Verification items for the finished model (mm, model axes). Face numbers are marked on the shaded views. Coordinates: 2 decimals unless noted, no trailing zeros. Order: outer loops, then holes, each group sorted by start corner. A loop starts at its lowest first (then second) coordinate and runs counter-clockwise, first axis right, second up. Notation, with made-up numbers: M 32.5,-1.75 L 83.5,-1.75 A21 ccw 83.5,15.25 Z; hole C 34,-37 d3. An arc over 180 degrees is marked long. Write item = value, one per line.
```python
from build123d import *

# Parameters (mm, degrees)
EXTRUDE_1_DEPTH     = 8
SKETCH_2_R          = 7.5
CUT_EXTRUDE_1_DEPTH = 10


with BuildPart() as part:
    # 草图1 → 凸台-拉伸1 (new body)
    with BuildSketch(Plane(origin=(0, 0, 0), x_dir=(0, 0, -1), z_dir=(1, 0, 0))):
        with BuildLine():
            ThreePointArc((15, 0), (0, 15), (-15, 0))
            Line((-15, 0), (-12.5, -200))
            ThreePointArc((-12.5, -200), (0, -212.5), (12.5, -200))
            Line((12.5, -200), (15, 0))
        make_face()
    extrude(amount=EXTRUDE_1_DEPTH)

    # 草图2 → 切除-拉伸1 (cut)
    with BuildSketch(Plane(origin=(8, 0, 0), x_dir=(0, 0, -1), z_dir=(1, 0, 0))):
        Circle(SKETCH_2_R)
        with Locations((0, -200)):
            Circle(SKETCH_2_R)
    extrude(amount=-CUT_EXTRUDE_1_DEPTH, mode=Mode.SUBTRACT)


solid = part.part
```
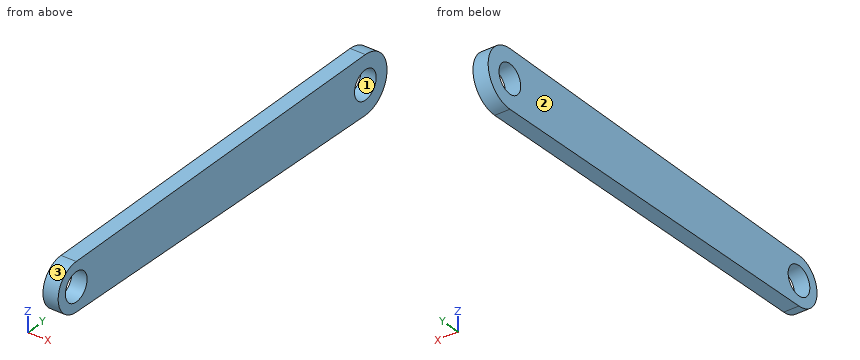
Item 1: Sectioned sample at B-B, the plane x = 6. Enter the section's corners in (y, z), then the cut area to 3 significant figures.
Report:
outline = M -200,-12.5 L 0,-15 A15 ccw 0,15 L -200,12.5 A12.5 ccw Z; hole C -200,0 d15; hole C 0,0 d15
area = 5,750 mm^2
Item 2: Release check for a two-part mould opening along Z. For the marked faces 1, 2 and 3 record: pulls with the +Z half, pulls with the -Z half, needs draft (parallel to the pull), parting line crosses it, or undercut.
Report:
face_1 = undercut
face_2 = needs draft
face_3 = parting line crosses it
Item 3: Sectioned sample at A-A, the plane z = 0. Enter the section's corners in (x, y), then the cut area to 3 significant figures.
Report:
outline = M 0,-212.5 L 8,-212.5 L 8,-207.5 L 0,-207.5 Z; M 0,-192.5 L 8,-192.5 L 8,-7.5 L 0,-7.5 Z; M 0,7.5 L 8,7.5 L 8,15 L 0,15 Z
area = 1,580 mm^2
Item 4: Sectioned sample at D-D, the plane y = -122.5. Enter the section's corners in (x, z).
Report:
outline = M 0,-13.47 L 8,-13.47 L 8,13.47 L 0,13.47 Z
Item 5: Scan lines: L1, parallel to Y at x = 6.5, z = 0; L2, parallel to Y at x = 1, z = 6.5; L3, parallel to Z at x = 4.5, y = -195.5. Record each from-to range of solid material in increasing order. Write a range as from..to.
Report:
L1 = -212.5..-207.5, -192.5..-7.5, 7.5..15
L2 = -210.68..-203.74, -196.26..-3.74, 3.74..13.52
L3 = -12.56..-6, 6..12.56
Item 6: Gauge pin test, flat ends, axial feed: pin 1 (1.5 mm diameter, centred on x = 2.5, y = -91, fed in from -Z); pin 2 (1 mm diameter, centred on x = 6.5, y = -141, fed in from -Z); pin 3 (2 mm diameter, centred on x = 6.5, z = -4, fed in from -Y). Record the tip position at first contact, or that the pin passes through.
Report:
pin_1 = -13.87
pin_2 = -13.24
pin_3 = -212.13
Item 7: Sectioned sample at C-C, the plane y = -37.5. Enter the section's corners in (x, z).
Report:
outline = M 0,-14.53 L 8,-14.53 L 8,14.53 L 0,14.53 Z
